Autodesk Inventor part; units mm, degrees
ref_plane "YZ Plane" through (0, 0, 0) normal (1, 0, 0) x (0, 1, 0)
ref_plane "XZ Plane" through (0, 0, 0) normal (0, 1, 0) x (-1, 0, 0)
ref_plane "XY Plane" through (0, 0, 0) normal (0, 0, 1) x (1, 0, 0)
sketch "Skizze1" plane through (0, 0, 0) normal (0, 0, 1) x (1, 0, 0)
  line L0 (0, 0) -> (45, 0)
  line L1 (45, 0) -> (0, 45)
  line L2 (0, 45) -> (0, 0)
  dimension "d0" = 45
  dimension "d1" = 45
extrude "Extrusion1" add sketch "Skizze1" along normal blind 4
sketch "Skizze4" plane through (0, 0, 4) normal (0, 0, 1) x (1, 0, 0)
  line L0 (45, 0) -> (0, 45)
  line L1 (45, 0) -> (45, -3.2)
  line L2 (45, -3.2) -> (-3.2, -3.2)
  line L3 (-3.2, -3.2) -> (-3.2, 45)
  line L4 (-3.2, 45) -> (0, 45)
  line L5 (0, 0) -> (45, 0)
  line L6 (0, 45) -> (0, 0)
  dimension "d20" = 3.2
  dimension "d21" = 3.2
extrude "Extrusion3" add sketch "Skizze4" against normal blind 16 contours L1 L2 L3 L4 L6 L5
sketch "Skizze2" plane through (0, 0, 4) normal (0, 0, 1) x (1, 0, 0)
  line L0 (45, 0) -> (0, 45)
  point P0 (0, 0)
  point P1 (8.565, 23)
  point P2 (23, 8.565)
  dimension "d11" = 9.5
  dimension "d12" = 9.5
  dimension "d14" = 22
  dimension "d15" = 22
hole "Bohrung1" at (8.565, 23, 4) at (23, 8.565, 4) direction (0, 0, -1) diameter 16 end through all
sketch "Skizze5" plane through (0, 0, 0) normal (0, 1, 0) x (1, 0, 0)
  line L0 (45, 0) -> (45, 12)
  line L1 (45, 0) -> (0, 0)
  point P0 (41, 6)
  dimension "d31" = 4
  dimension "d32" = 6
hole "Bohrung2" at (41, 0, -6) direction (0, -1, 0) diameter 3.5 end through all counterbore diameter 6 counterbore depth 2
sketch "Skizze6" plane through (0, 0, 0) normal (1, 0, 0) x (0, 0, -1)
  line L0 (0, 0) -> (0, 45)
  line L1 (0, 45) -> (12, 45)
  point P0 (6, 41)
  dimension "d40" = 6
  dimension "d41" = 4
hole "Bohrung3" at (0, 41, -6) direction (-1, 0, 0) diameter 3.5 end through all counterbore diameter 6 counterbore depth 2
equation "\"d0\" = d1"
equation "\"d21\" = d20"
properties part number "Buttons_Mount_v1"
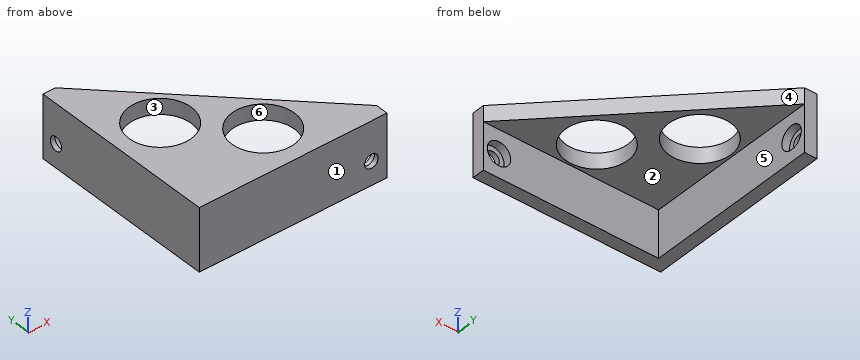
Could you check a few things on this model? Use its own coordinates, in mm. Face numbers are marked on the shaded views. A direction names the side the tool comes from. Round coordinates to 2 decimals unless told otherwise and drop trailing zeros. Loops run counter-clockwise (first coordinate to the right, second up) from the corner with the lowest first, then second, coordinate; pieces in that order, holes last. Notation, with made-up numbers: M 19.5,83.25 L 46.5,83.25 A24 cw 46.5,102.25 Z; hole C 71,3.5 d10. An arc over 180 degrees is marked long. Answer as CSV lines item,"result".
1) Imagine slicing it at D-D on y = 35. List the corners of the cut face in (x, z) for me, and give its area (3 significant figures).
From the geometry:
outline,"M -3.2,-12 L 0,-12 L 0,0 L 10,0 L 10,4 L -3.2,4 Z"
area,"91.2 mm^2"
2) Imagine slicing it at C-C on z = -5. List the corners of the cut face in (x, y) for me, and give its area (3 significant figures).
From the geometry:
outline,"M -3.2,-3.2 L 39.56,-3.2 L 39.56,-2 L 38.17,-2 L 38.17,0 L 0,0 L 0,38.17 L -2,38.17 L -2,39.56 L -3.2,39.56 Z; M -3.2,42.44 L -2,42.44 L -2,43.83 L 0,43.83 L 0,45 L -3.2,45 Z; M 42.44,-3.2 L 45,-3.2 L 45,0 L 43.83,0 L 43.83,-2 L 42.44,-2 Z"
area,"269 mm^2"
3) We'd pull the mould along Y, two halves only. Please class the marked faces 3, 4, 5 and 6: released by +Y, released by -Y, zero draft, split by the parting line, or undercut.
From the geometry:
face 3,"undercut"
face 4,"released by +Y"
face 5,"zero draft"
face 6,"undercut"
4) If I drill on probe 1 along X at (y, z) = (-2.9, -6); probe 2 along Z at (x, y) = (41, -2.7); probe 3 along Z at (x, y) = (-1.5, 41), over which ranges is the centre line in solid material (lowest first)?
From the geometry:
probe 1,"-3.2 to 39.25, 42.75 to 45"
probe 2,"-12 to -7.75, -4.25 to 4"
probe 3,"-12 to -9, -3 to 4"
5) For pin 1 Ø3 at (x, z) = (41.5, -5) entering from +Y; pin 2 Ø8 at (x, z) = (39.5, 0) entering from +Y; pin 3 Ø5 at (y, z) = (41, -6) entering from +X; pin 4 Ø3 at (y, z) = (41, -6) entering from +X, each with a flat end and sliding along its axis, tell me the tip position at first contact or that it passes through.
From the geometry:
pin 1,"y = -2"
pin 2,"y = 9.5"
pin 3,"x = -2"
pin 4,"through"
6) Which directions (+Z, -Z, +X, -X, +Y, -Y) give clear straight access to the entire face, cutting with the end or side of a thin tool? Please do the marked faces 1 and 2.
From the geometry:
face 1,"+Z, -Z, +X, -X, -Y"
face 2,"-Z, +X, +Y"
7) Imagine slicing it at B-B on y = 41. List the corners of the cut face in (x, z) for me.
From the geometry:
outline,"M -3.2,-12 L 0,-12 L 0,-9 L -2,-9 L -2,-7.75 L -3.2,-7.75 Z; M -3.2,-4.25 L -2,-4.25 L -2,-3 L 0,-3 L 0,0 L 4,0 L 4,4 L -3.2,4 Z"
8) Imagine slicing it at A-A on x = 23. List the corners of the cut face in (y, z) for me (3 decimals).
From the geometry:
outline,"M -3.2,-12 L 0,-12 L 0,0 L 0.565,0 L 0.565,4 L -3.2,4 Z; M 16.565,0 L 22,0 L 22,4 L 16.565,4 Z"
